Geometry check sheet. Reference: the model listing, model coordinates, mm. A direction names the side the tool comes from. Coordinates: 2 decimals unless noted, no trailing zeros. Write each loop counter-clockwise with the first axis right and the second up, starting at its lowest first coordinate (ties: lowest second). Pieces come first, ordered by that corner, then holes. Notation, with made-up numbers: (72.5, 43) - (129.5, 43) arc R15 ccw to (129.5, 55) - close; hole circle Ø10 at (38, 70). An arc over 180 degrees is marked (long way). Answer as a JSON object with one key per item and string values. Group by question number.
from build123d import *

# Parameters (mm, degrees)
F0_W     = 145.7543373108
F0_H     = 101.455360651
F1_DEPTH = 101.6
F4_DEPTH = 25.4
F5_R     = 27.7028558339
F6_DEPTH = 127
F7_R     = 9.4879740748
F7_R_2   = 9.6289901624
F8_DEPTH = 152.4


with BuildPart() as f1:
    # F0 (on Front) → F1 (new body)
    with BuildSketch(Plane.XZ):
        Rectangle(F0_W, F0_H)
    extrude(amount=F1_DEPTH)

    # F3 (on face) + F2 (on face) → F4 (join)
    with BuildSketch(Plane.XY.offset(50.7276803255)):
        with BuildLine():
            Line((-45.8042988354, -101.6), (45.8042988354, -101.6))
            ThreePointArc((45.8042988354, -101.6), (0, -55.7957011646), (-45.8042988354, -101.6))
        make_face()
    with BuildSketch(Plane(origin=(0, 0, -50.7276803255), x_dir=(1, 0, 0), z_dir=(0, 0, -1))):
        with BuildLine():
            ThreePointArc((-46.1219863385, 101.6), (0, 55.4780136615), (46.1219863385, 101.6))
            Line((46.1219863385, 101.6), (-46.1219863385, 101.6))
        make_face()
    extrude(amount=F4_DEPTH, dir=(0, 0, 1))

    # F5 (on face) → F6 (cut)
    with BuildSketch(Plane(origin=(0, 0, -50.7276803255), x_dir=(1, 0, 0), z_dir=(0, 0, -1))):
        with Locations((0, 101.6)):
            Circle(F5_R)
    extrude(amount=-F6_DEPTH, mode=Mode.SUBTRACT)

    # F7 (on face) → F8 (cut)
    with BuildSketch(Plane.XZ.offset(101.6)):
        with Locations((-57.1189150214, 0)):
            Circle(F7_R)
        with Locations((59.1401457787, 0)):
            Circle(F7_R_2)
    extrude(amount=-F8_DEPTH, mode=Mode.SUBTRACT)


solid = f1.part
(1) Draft check along Z on faces 1 (the face through (-1, -50, -50.728)), 2 (the face through (-64.65, -51.51, -5.77)), 3 (the face through (-72.877, -50, -1)). Enter one of: +Z half, -Z half, draft (parallel to the pull), parting line (faces both ways), or undercut.
(2) Set-up check for faces 4 (the face through (-0.609, -73.904, 11.812)), 5 (the face through (1.007, -55.807, 63.25)): record each of +Z, -Z, +X, -X, +Y, -Y from which the full face is reachable in a straight line by a thin tool's end or side.
(3) Section check C-C (x = 0). Record the cut outline in (y, z).
(4) Section check D-D (y = -16). Record the cut outline in (x, z), and give its area (3 significant figures).
(5) Section check B-B (z = 0). Record the cut outline in (x, y), and give its area (3 significant figures).
(6) Gauge pin test, flat ends, axial feed: pin 1 (8 mm diameter, centred on x = 3.5, z = -8, fed in from -Y); pin 2 (2 mm diameter, centred on x = 58, y = -26, fed in from +Z); pin 3 (15 mm diameter, centred on x = -57.12, z = 0, fed in from -Y); pin 4 (1.5 mm diameter, centred on x = 17, z = 11, fed in from +Y). Record the tip position at first contact, or that the pin passes through.
(7) Material ranges on L1, parallel to X at y = -16.5, z = -1.5; L2, parallel to Z at x = -38.5, y = -69; L3, parallel to Z at x = -54, y = -42, recorded low to high. Write a range as [from, to].
(8) Section check A-A (y = -92.5). Record the cut outline in (x, z), and give its area (3 significant figures).
Conclusion:
{
 "1": {"face 1": "-Z half", "face 2": "undercut", "face 3": "draft"},
 "2": {"face 4": "+Z, -Z, -Y", "face 5": "+Z, +Y"},
 "3": {"outline": "(-73.9, -50.73) - (0, -50.73) - (0, 50.73) - (-55.8, 50.73) - (-55.8, 76.13) - (-73.9, 76.13) - close"},
 "4": {"outline": "(-72.88, -50.73) - (72.88, -50.73) - (72.88, 50.73) - (-72.88, 50.73) - close; hole circle Ø18.98 at (-57.12, 0); hole circle Ø19.26 at (59.14, 0)", "area": "14,200 mm^2"},
 "5": {"outline": "(-72.88, -101.6) - (-66.61, -101.6) - (-66.61, 0) - (-72.88, 0) - close; (-47.63, -101.6) - (-27.7, -101.6) arc R27.7 cw to (27.7, -101.6) - (49.51, -101.6) - (49.51, 0) - (-47.63, 0) - close; (68.77, -101.6) - (72.88, -101.6) - (72.88, 0) - (68.77, 0) - close", "area": "9,720 mm^2"},
 "6": {"pin 1": "stops at y = -74.93", "pin 2": "stops at z = 50.73", "pin 3": "passes through", "pin 4": "stops at y = 0"},
 "7": {"L1": "x = [-72.88, -66.49], [-47.75, 49.63], [68.65, 72.88]", "L2": "z = [-50.73, 50.73]", "L3": "z = [-50.73, -8.96], [8.96, 50.73]"},
 "8": {"outline": "(-72.88, -50.73) - (-26.17, -50.73) - (-26.17, 76.13) - (-44.89, 76.13) - (-44.89, 50.73) - (-72.88, 50.73) - close; (26.17, -50.73) - (72.88, -50.73) - (72.88, 50.73) - (44.89, 50.73) - (44.89, 76.13) - (26.17, 76.13) - close; hole circle Ø18.98 at (-57.12, 0); hole circle Ø19.26 at (59.14, 0)", "area": "9,860 mm^2"}
}
